Design review of the part built by this model. Coordinates are the model's own, in mm. A direction names the side the tool comes from. Give positions to 0.01 mm unless a question says otherwise; leave off trailing zeros. Loops run counter-clockwise (first coordinate to the right, second up) from the corner with the lowest first, then second, coordinate; pieces in that order, holes last.
from build123d import *
from OCP.BRepFilletAPI import BRepFilletAPI_MakeChamfer

# Parameters (mm, degrees)
BOSS_EXTRUDE1_DEPTH = 15
SKETCH2_R           = 2
CUT_EXTRUDE1_DEPTH  = 52.967393623
SKETCH3_R           = 2
CUT_EXTRUDE2_DEPTH  = 3.5
CHAMFER1_SIZE       = 2.5
CHAMFER1_SIZE2      = 1.750518846
CHAMFER2_SIZE       = 2.5
CHAMFER2_SIZE2      = 1.750518846
FILLET1_R           = 5
FILLET2_R           = 1.5
FILLET3_R           = 1
FILLET4_R           = 4.5


with BuildPart() as part:
    # Sketch1 → Boss-Extrude1 (new body)
    with BuildSketch(Plane.XY):
        with BuildLine():
            Line((24.6, 0), (38.1, 0))
            Line((38.1, 0), (38.1, -3.5))
            Line((38.1, -3.5), (27.318446602, -3.5))
            Line((27.318446602, -3.5), (22.893526956, -20.825415956))
            ThreePointArc((22.893526956, -20.825415956), (-8.755509301, -30.749473973), (-3.5, 2))
            Line((-3.5, 2), (-3.5, 19.491933385))
            Line((-3.5, 19.491933385), (0, 19.491933385))
            Line((0, 19.491933385), (0, -0.508066615))
            ThreePointArc((0, -0.508066615), (-7.298847951, -27.328549553), (19.502381092, -19.959315656))
            Line((19.502381092, -19.959315656), (24.6, 0))
        make_face()
    extrude(amount=BOSS_EXTRUDE1_DEPTH)

    # Sketch2 → Cut-Extrude1 (cut, through all)
    with BuildSketch(Plane.XZ.offset(3.5)):
        with Locations(Location((32.318446602, 7.5, 0), (0, 0, 270))):
            Circle(SKETCH2_R)
    extrude(amount=-CUT_EXTRUDE1_DEPTH, mode=Mode.SUBTRACT)

    # Sketch3 → Cut-Extrude2 (cut)
    with BuildSketch(Plane.ZY.offset(3.5)):
        with Locations(Location((7.5, 11.491933385, 0), (0, 0, 270))):
            Circle(SKETCH3_R)
    extrude(amount=-CUT_EXTRUDE2_DEPTH, mode=Mode.SUBTRACT)

    # Chamfer1: one chamfer whose edges measure the first distance from different faces: ONE call of the kernel's chamfer builder (chamfer() names one face for all edges)
    chamfer1_edges_1 = [part.edges().sort_by_distance(p)[0] for p in [
        (32.318446602, -3.5, 9.5),
    ]]
    chamfer1_side_1 = [part.faces().sort_by_distance(p)[0] for p in [
        (37.915272662, -3.5, 7.5),
    ]]
    chamfer1_edges_2 = [part.edges().sort_by_distance(p)[0] for p in [
        (-3.5, 13.491933385, 7.5),
    ]]
    chamfer1_side_2 = [part.faces().sort_by_distance(p)[0] for p in [
        (-3.5, 2.230427371, 7.5),
    ]]
    chamfer1 = BRepFilletAPI_MakeChamfer(part.part.solid().wrapped)
    for e in chamfer1_edges_1:
        chamfer1.Add(CHAMFER1_SIZE, CHAMFER1_SIZE2, e.wrapped, chamfer1_side_1[0].wrapped)  # the first distance lies on this face
    for e in chamfer1_edges_2:
        chamfer1.Add(CHAMFER1_SIZE, CHAMFER1_SIZE2, e.wrapped, chamfer1_side_2[0].wrapped)  # the first distance lies on this face
    add(Compound.cast(chamfer1.Shape()), mode=Mode.REPLACE)

    # Chamfer2: one chamfer whose edges measure the first distance from different faces: ONE call of the kernel's chamfer builder (chamfer() names one face for all edges)
    chamfer2_edges_1 = [part.edges().sort_by_distance(p)[0] for p in [
        (-1.75, 19.491933385, 0),
        (38.1, -1.75, 0),
    ]]
    chamfer2_side_1 = [part.faces().sort_by_distance(p)[0] for p in [
        (-2.732075997, 10.745966692, 0),
    ]]
    chamfer2_edges_2 = [part.edges().sort_by_distance(p)[0] for p in [
        (-1.75, 19.491933385, 15),
    ]]
    chamfer2_side_2 = [part.faces().sort_by_distance(p)[0] for p in [
        (-1.75, 19.491933385, 7.5),
    ]]
    chamfer2_edges_3 = [part.edges().sort_by_distance(p)[0] for p in [
        (38.1, -1.75, 15),
    ]]
    chamfer2_side_3 = [part.faces().sort_by_distance(p)[0] for p in [
        (38.1, -1.75, 7.5),
    ]]
    chamfer2 = BRepFilletAPI_MakeChamfer(part.part.solid().wrapped)
    for e in chamfer2_edges_1:
        chamfer2.Add(CHAMFER2_SIZE, CHAMFER2_SIZE2, e.wrapped, chamfer2_side_1[0].wrapped)  # the first distance lies on this face
    for e in chamfer2_edges_2:
        chamfer2.Add(CHAMFER2_SIZE, CHAMFER2_SIZE2, e.wrapped, chamfer2_side_2[0].wrapped)  # the first distance lies on this face
    for e in chamfer2_edges_3:
        chamfer2.Add(CHAMFER2_SIZE, CHAMFER2_SIZE2, e.wrapped, chamfer2_side_3[0].wrapped)  # the first distance lies on this face
    add(Compound.cast(chamfer2.Shape()), mode=Mode.REPLACE)

    # Fillet1
    fillet1_edges = [part.edges().sort_by_distance(p)[0] for p in [
        (0, -0.508066615, 7.5),
    ]]
    fillet(fillet1_edges, radius=FILLET1_R)

    # Fillet2
    fillet2_edges = [part.edges().sort_by_distance(p)[0] for p in [
        (-3.5, 2, 7.5),
    ]]
    fillet(fillet2_edges, radius=FILLET2_R)

    # Fillet3
    fillet3_edges = [part.edges().sort_by_distance(p)[0] for p in [
        (27.318446602, -3.5, 7.5),
    ]]
    fillet(fillet3_edges, radius=FILLET3_R)

    # Fillet4
    fillet4_edges = [part.edges().sort_by_distance(p)[0] for p in [
        (24.6, 0, 7.5),
    ]]
    fillet(fillet4_edges, radius=FILLET4_R)


solid = part.part
Q1. Take a section at D-D (z = 13.5). Give the boundary of the cut face in (x, y), plus the area to 3 significant figures.
Results:
outline: (-4.36, 1.62) arc R19.5 ccw (long way) to (22.89, -20.83) - (27.13, -4.25) arc R1 cw to (28.1, -3.5) - (37.4, -3.5) - (37.4, 0) - (28.1, 0) arc R4.5 ccw to (23.74, -3.39) - (19.5, -19.96) arc R16 cw (long way) to (-2.86, -1.54) arc R5 ccw to (0, 2.97) - (0, 18.79) - (-3.5, 18.79) - (-3.5, 2.97) arc R1.5 cw to start
area: 423 mm2
Q2. Take a section at A-A (y = -16). Give the boundary of the cut face in (x, z), plus the area to 3 significant figures.
Results:
outline: (-15.5, 0) - (-12, 0) - (-12, 15) - (-15.5, 15) - close; (20.51, 0) - (24.13, 0) - (24.13, 15) - (20.51, 15) - close
area: 107 mm2
Q3. Draft analysis for pull direction Y (two halves, no side actions). For faces 1 (the face through (-0.887, 9.584, 8.101)), 2 (the face through (-7.969, -31.395, 7.395)), 3 (the face through (-0.795, 0.268, 7.605)), 4 (the face through (31.101, -0.887, 9.087)), state which applies: pulls with the +Y half, pulls with the -Y half, needs draft (parallel to the pull), parting line crosses it, or undercut.
Results:
face 1: undercut
face 2: parting line crosses it
face 3: undercut
face 4: needs draft
Q4. Insertion check: pin 1 (6.5 mm diameter, centred on y = 11.49, z = 7.5, fed in from +X); pin 2 (3 mm diameter, centred on x = 32.5, z = 6, fed in from +Y); pin 3 (12 mm diameter, centred on x = -1, y = -14.5, fed in from -Z); pin 4 (1.5 mm diameter, centred on x = 1.5, z = 4.5, fed in from +Y). Each pin has a flat end and moves straight along its axis. Give the tip position at first contact, or say it passes through.
Results:
pin 1: stops at x = 0
pin 2: stops at y = 0
pin 3: passes through
pin 4: stops at y = -31.67
Q5. Take a section at C-C (z = 7.5). Give the number of separate pieces and of enclosed holes in the cut face, plus the area to 3 significant figures.
Results:
separate pieces: 3
enclosed holes: 0
area: 391 mm2
Q6. Wall thickness on line 1 (X direction, y = -0.5, z = 7.5); line 2 (X direction, y = -0.95, z = 7.5); line 3 (Y direction, x = 30, z = 1.75): over which ranges is each line inside the solid? List them lowest first.
Results:
line 1: x = -7.83 to -1.4, 26.03 to 30.32, 34.32 to 38.1
line 2: x = -8.4 to -1.9, 25.33 to 30.32, 34.32 to 38.1
line 3: y = -3.5 to 0
Q7. Take a section at B-B (x = -1). Give the boundary of the cut face in (y, z).
Results:
outline: (-34.85, 0) - (-31.2, 0) - (-31.2, 15) - (-34.85, 15) - close; (-0.03, 0) - (16.99, 0) - (19.49, 1.75) - (19.49, 12.5) - (17.74, 15) - (-0.03, 15) - close; hole circle Ø4 at (11.49, 7.5)
Q8. Tool access review of faces 5 (the face through (37, -3.5, 6)), 6 (the face through (25.37, -0.92, 7.6)), 7 (the face through (-3.5, 7, 11)), 8 (the face through (-3, -1, 0)), 9 (the face through (0, 9.5, 5.7)): name each direction out of +Z, -Z, +X, -X, +Y, -Y from which nothing blocks a thin tool from reaching the whole face with its end or side.
Results:
face 5: +Z, -Z, +X, -Y
face 6: +Z, -Z, +Y
face 7: +Z, -Z, -X, +Y
face 8: -Z, +X, -X, +Y, -Y
face 9: +Z, -Z, +X, +Y
